Here's how the part is built. I have some questions about the finished solid (model axes, mm). A direction names the side the tool comes from. Coordinates: 2 decimals unless noted, no trailing zeros. Write each loop counter-clockwise with the first axis right and the second up, starting at its lowest first coordinate (ties: lowest second). Pieces come first, ordered by that corner, then holes.
```python
from build123d import *


with BuildPart() as part:
    # Sketch1 → Revolve1 (revolve)
    with BuildSketch(Plane(origin=(0, 0, 0), x_dir=(1, 0, 0), z_dir=(0, 1, 0))):
        with BuildLine():
            Line((0, 0), (0, 1.016))
            Line((0, 1.016), (12.7, 1.016))
            Line((12.7, 1.016), (12.7, 1.27))
            Line((12.7, 1.27), (19.05, 1.27))
            ThreePointArc((19.05, 1.27), (19.396522774, 1.335269355), (19.695555117, 1.522132353))
            ThreePointArc((19.695555117, 1.522132353), (20.074329418, 1.758825483), (20.513258265, 1.8415))
            Line((20.513258265, 1.8415), (33.213258265, 1.8415))
            Line((33.213258265, 1.8415), (33.213258265, 1.5875))
            Line((33.213258265, 1.5875), (20.513258265, 1.5875))
            ThreePointArc((20.513258265, 1.5875), (20.166735491, 1.522230645), (19.867703148, 1.335367647))
            ThreePointArc((19.867703148, 1.335367647), (19.488928847, 1.098674517), (19.05, 1.016))
            Line((19.05, 1.016), (20.513258265, 1.016))
            Line((20.513258265, 1.016), (20.513258265, 0.635))
            Line((20.513258265, 0.635), (25.593258265, 0.635))
            Line((25.593258265, 0.635), (25.593258265, 0))
            Line((25.593258265, 0), (0, 0))
        make_face()
    revolve(axis=Axis((25.593258265, 0, 0), (-1, 0, 0)))


solid = part.part
```
1) On a 3-axis mill with a long thin cutter (end or side, diameter ignored), from which of +Z, -Z, +X, -X, +Y, -Y can I reach the whole of each face in a straight line? I mean faces 1 (the face through (26.952, 1.634, -0.85)), 2 (the face through (26.77, 1.55, 0.34)), 3 (the face through (6.44, 0.99, 0.22)). Say none if no direction works.
Values follow:
face 1: +X, -X
face 2: +X
face 3: -X
2) I need wall thicknesses on probe 1 along Y at (x, z) = (25.25, 0) (1 decimal); probe 2 along Y at (x, z) = (30, 0). Which ranges of each line are inside material? Lowest first, please.
Values follow:
probe 1: y = -1.8 to -1.6, -0.6 to 0.6, 1.6 to 1.8
probe 2: y = -1.84 to -1.59, 1.59 to 1.84
3) Imagine slicing it at A-A on x = 22.5. Please give me the cut outline in (y, z) (1 decimal), then the cut area to 3 significant figures.
Values follow:
outline: circle Ø3.7 at (0, 0); circle Ø1.3 at (0, 0); hole circle Ø3.2 at (0, 0)
area: 4.00 mm2
4) Imagine slicing it at D-D on x = 14.5. Please give me the cut outline in (y, z), then the cut area to 3 significant figures.
Values follow:
outline: circle Ø2.54 at (0, 0)
area: 5.07 mm2
5) Imagine slicing it at C-C on x = 8.5. Please give me the cut outline in (y, z), then the cut area to 3 significant figures.
Values follow:
outline: circle Ø2.03 at (0, 0)
area: 3.24 mm2
6) Will these pins go through, and if not, where does the flat tip stop? pin 1 (1 mm diameter, centred on x = 12, y = -0.5, fed in from +Z); pin 2 (0.6 mm diameter, centred on y = -0.5, z = 0, fed in from +X).
Values follow:
pin 1: stops at z = 1.02
pin 2: stops at x = 25.59
7) Imagine slicing it at B-B on x = 29. Please give me the cut outline in (y, z) (1 decimal).
Values follow:
outline: circle Ø3.7 at (0, 0); hole circle Ø3.2 at (0, 0)
8) We'd pull the mould along Z, two halves only. Please class faces 4 (the face through (0, 0, 0)), 5 (the face through (23.09, -0.63, 0.08)), 6 (the face through (15.92, -1.26, 0.17)), 7 (the face through (25.593, 0, 0)): pulls with the +Z half, pulls with the -Z half, needs draft (parallel to the pull), parting line crosses it, or undercut.
Values follow:
face 4: needs draft
face 5: undercut
face 6: parting line crosses it
face 7: undercut
